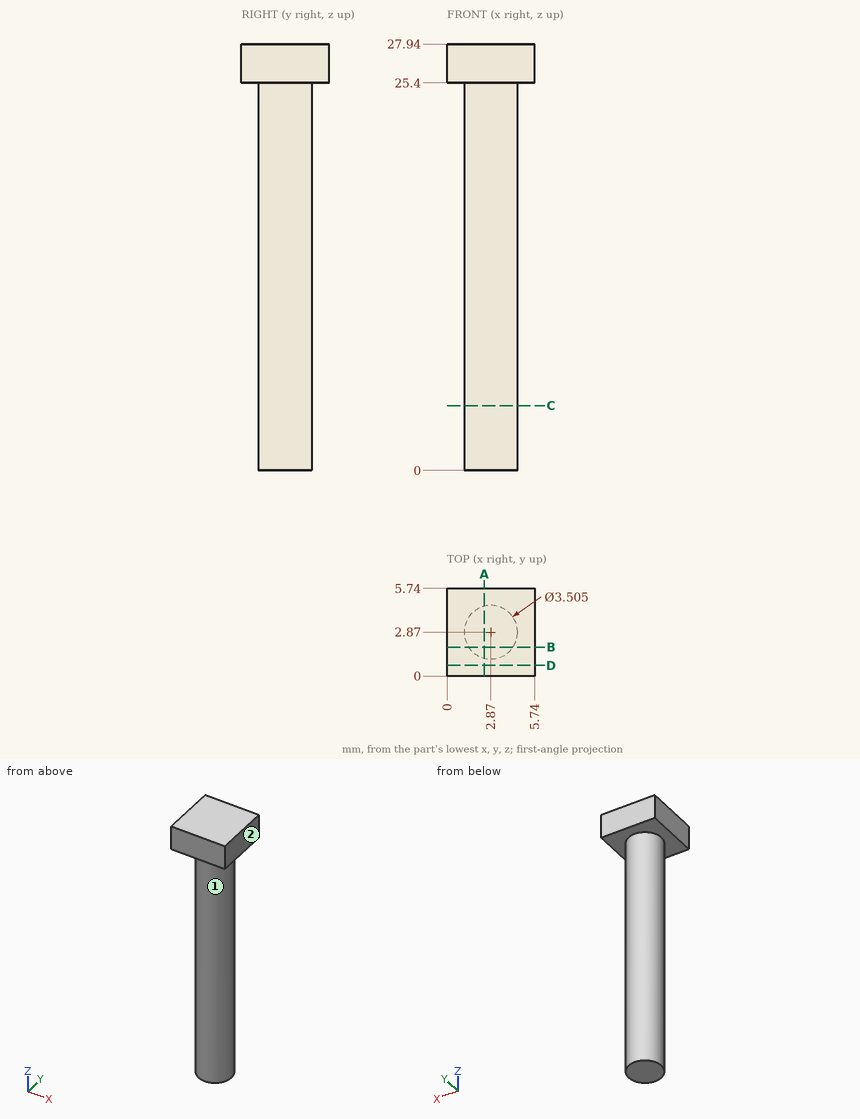
Input: dimensioned drawing with shaded views. Units: mm. Origin: part minimum x, y, z. A direction names the side the tool comes from. Coordinates: 2 decimals unless noted, no trailing zeros. Write each loop counter-clockwise with the first axis right and the second up, starting at its lowest first coordinate (ties: lowest second). Pieces come first, ordered by that corner, then holes. Notation, with made-up numbers: M -10,-24.5 L 16,-24.5 A23 cw 16,11.5 Z; hole C -25.75,74.5 d1. An arc over 180 degrees is marked long. Answer as a JSON object with one key per item and string values. Group by question number.
(1) Set-up query: the marked faces 1 and 2. Return all of +Z, -Z, +X, -X, +Y, -Y with unobstructed straight access to the full face (end or side cutting, diameter ignored); none if empty.
(2) Section B-B on y = 1.9. Output: boundary loops of the cut face in (x, z).
(3) Section A-A on x = 2.45. Output: boundary loops of the cut face in (y, z).
(4) Section D-D on y = 0.7. Output: boundary loops of the cut face in (x, z).
(5) Ray query, line 1 along Z through (x, y) = (0.75, 0.85); line 2 along Y through (x, z) = (3.1, 15); line 3 along X through (y, z) = (2.3, 24). Return the intervals inside material, ascending. Write a range as [from, to].
(6) Contact query for flat-ended pins moving along their axis: P1, Ø1.5, axis at y = 4, z = 7.5, coming from the +X side; P2, Ø1.5, axis at x = 4, z = 3.5, coming from the +Y side. Output: stop coordinate, or through.
(7) Section C-C on z = 4.25. Output: boundary loops of the cut face in (x, y) (1 decimal).
Result set:
{
 "1": {"face 1": "-Z", "face 2": "+Z, -Z, +X, +Y, -Y"},
 "2": {"outline": "M 0,25.4 L 1.41,25.4 L 1.41,0 L 4.33,0 L 4.33,25.4 L 5.74,25.4 L 5.74,27.94 L 0,27.94 Z"},
 "3": {"outline": "M 0,25.4 L 1.17,25.4 L 1.17,0 L 4.57,0 L 4.57,25.4 L 5.74,25.4 L 5.74,27.94 L 0,27.94 Z"},
 "4": {"outline": "M 0,25.4 L 5.74,25.4 L 5.74,27.94 L 0,27.94 Z"},
 "5": {"line 1": "z = [25.4, 27.94]", "line 2": "y = [1.13, 4.61]", "line 3": "x = [1.21, 4.53]"},
 "6": {"P1": "stops at x = 4.58", "P2": "stops at y = 4.58"},
 "7": {"outline": "C 2.9,2.9 d3.5"}
}
